Geometry: final body of the model. Coordinates: model frame, mm. A direction names the side the tool comes from. Round coordinates to 2 decimals unless told otherwise and drop trailing zeros. Loops run counter-clockwise (first coordinate to the right, second up) from the corner with the lowest first, then second, coordinate; pieces in that order, holes last. Notation, with made-up numbers: (36, -12.5) - (78, -12.5) arc R8 cw to (78, 0.5) - close; hole circle Ø1 at (48, 87). An arc over 180 degrees is marked (long way). Answer as CSV lines item,"result".
from build123d import *

# Parameters (mm, degrees)
BOSS_EXTRUDE1_DEPTH = 6
SKETCH2_R           = 1.25
CUT_EXTRUDE1_DEPTH  = 10
FILLET1_R           = 1
FILLET2_R           = 0.5
FILLET3_R           = 2.5


with BuildPart() as part:
    # Sketch1 → Boss-Extrude1 (new body)
    with BuildSketch(Plane.XY):
        with BuildLine():
            Line((-3.092329219, 1), (-9.531128874, 1))
            Line((-9.531128874, 1), (-9.531128874, 3))
            Line((-9.531128874, 3), (-4.031128874, 3))
            ThreePointArc((-4.031128874, 3), (0, 5.5), (4.031128874, 3))
            Line((4.031128874, 3), (9.531128874, 3))
            Line((9.531128874, 3), (9.531128874, 1))
            Line((9.531128874, 1), (3.092329219, 1))
            ThreePointArc((3.092329219, 1), (0, 3.25), (-3.092329219, 1))
        make_face()
    extrude(amount=BOSS_EXTRUDE1_DEPTH)

    # Sketch2 → Cut-Extrude1 (cut)
    with BuildSketch(Plane(origin=(0, 3, 0), x_dir=(1, 0, 0), z_dir=(0, 1, 0))):
        with Locations(Location((-6.5, -3, 0), (0, 0, 270))):
            Circle(SKETCH2_R)
        with Locations(Location((6.5, -3, 0), (0, 0, 270))):
            Circle(SKETCH2_R)
    extrude(amount=-CUT_EXTRUDE1_DEPTH, mode=Mode.SUBTRACT)

    # Fillet1
    fillet1_edges = [part.edges().sort_by_distance(p)[0] for p in [
        (-4.031128874, 3, 3),
        (4.031128874, 3, 3),
    ]]
    fillet(fillet1_edges, radius=FILLET1_R)

    # Fillet2
    fillet2_edges = [part.edges().sort_by_distance(p)[0] for p in [
        (-9.531128874, 1, 3),
        (-9.531128874, 3, 3),
        (9.531128874, 3, 3),
        (9.531128874, 1, 3),
    ]]
    fillet(fillet2_edges, radius=FILLET2_R)

    # Fillet3
    fillet3_edges = [part.edges().sort_by_distance(p)[0] for p in [
        (-3.092329219, 1, 3),
        (3.092329219, 1, 3),
    ]]
    fillet(fillet3_edges, radius=FILLET3_R)


solid = part.part
(1) Section A-A (x = -7.5). Output: boundary loops of the cut face in (y, z), and give its area (3 significant figures).
Findings below:
outline,"(1, 0) - (3, 0) - (3, 2.25) - (1, 2.25) - close; (1, 3.75) - (3, 3.75) - (3, 6) - (1, 6) - close"
area,"9.00 mm2"
(2) Section B-B (z = 3). Output: boundary loops of the cut face in (x, y), and give its area (3 significant figures).
Findings below:
outline,"(-9.53, 1.5) arc R0.5 ccw to (-9.03, 1) - (-7.75, 1) - (-7.75, 3) - (-9.03, 3) arc R0.5 ccw to (-9.53, 2.5) - close; (-5.25, 1) - (-4.56, 1) arc R2.5 ccw to (-2.58, 1.98) arc R3.25 cw to (2.58, 1.98) arc R2.5 ccw to (4.56, 1) - (5.25, 1) - (5.25, 3) - (4.61, 3) arc R1 cw to (3.77, 3.45) arc R4.5 ccw to (-3.77, 3.45) arc R1 cw to (-4.61, 3) - (-5.25, 3) - close; (7.75, 1) - (9.03, 1) arc R0.5 ccw to (9.53, 1.5) - (9.53, 2.5) arc R0.5 ccw to (9.03, 3) - (7.75, 3) - close"
area,"31.6 mm2"
(3) Section D-D (z = 5.45). Output: boundary loops of the cut face in (x, y), and give its area (3 significant figures).
Findings below:
outline,"(-9.53, 1.5) arc R0.5 ccw to (-9.03, 1) - (-4.56, 1) arc R2.5 ccw to (-2.58, 1.98) arc R3.25 cw to (2.58, 1.98) arc R2.5 ccw to (4.56, 1) - (9.03, 1) arc R0.5 ccw to (9.53, 1.5) - (9.53, 2.5) arc R0.5 ccw to (9.03, 3) - (4.61, 3) arc R1 cw to (3.77, 3.45) arc R4.5 ccw to (-3.77, 3.45) arc R1 cw to (-4.61, 3) - (-9.03, 3) arc R0.5 ccw to (-9.53, 2.5) - close"
area,"41.6 mm2"
(4) Access query for faces 1 (the face through (3.442, 1.265, 3.042)), 2 (the face through (-8, 3, 3)), 3 (the face through (8, 3, 3)). Directions: +Z, -Z, +X, -X, +Y, -Y. A direction counts if a zero-diameter tool reaches every point of the face in a straight line with its end or side. Return the directions, or none.
Findings below:
face 1,"+Z, -Z, -Y"
face 2,"+Z, -Z, -X, +Y"
face 3,"+Z, -Z, +X, +Y"
(5) Draft query along Z for faces 4 (the face through (0, 4, 0)), 5 (the face through (-9.531, 2, 3)), 6 (the face through (5.391, 2.014, 3.577)). Return one class per face: pulls with the +Z half, pulls with the -Z half, needs draft (parallel to the pull), parting line crosses it, or undercut.
Findings below:
face 4,"pulls with the -Z half"
face 5,"needs draft"
face 6,"undercut"
(6) Section C-C (x = 6.5). Output: boundary loops of the cut face in (y, z).
Findings below:
outline,"(1, 0) - (3, 0) - (3, 1.75) - (1, 1.75) - close; (1, 4.25) - (3, 4.25) - (3, 6) - (1, 6) - close"
(7) Pin query (flat end, axial travel): P1, Ø2, axis at x = -6.5, z = 3, coming from the +Y side; P2, Ø2, axis at x = -1.5, z = 3.5, coming from the -Y side; P3, Ø2, axis at x = 6.5, z = 4, coming from the +Y side. Return the tip coordinate at first contact, or that it passes through.
Findings below:
P1,"through"
P2,"y = 2.08"
P3,"y = 3"
(8) Material intervals for line 1 along X through (y, z) = (1.9, 3); line 2 along X through (y, z) = (2.65, 3.4); line 3 along X through (y, z) = (1.35, 1.15), sorted ascending.
Findings below:
line 1,"-9.53 to -7.75, -5.25 to -2.64, 2.64 to 5.25, 7.75 to 9.53"
line 2,"-9.51 to -7.68, -5.32 to -1.88, 1.88 to 5.32, 7.68 to 9.51"
line 3,"-9.51 to -3.29, 3.29 to 9.51"
